Verification items for the finished model (mm, model axes). Face numbers are marked on the shaded views. A direction names the side the tool comes from. Give positions to 0.01 mm unless a question says otherwise; leave off trailing zeros. Order: outer loops, then holes, each group sorted by start corner. A loop starts at its lowest first (then second) coordinate and runs counter-clockwise, first axis right, second up. Notation, with made-up numbers: (-36.5, 56) -> (4.5, 56) arc R22 ccw to (4.5, 83) -> close; hole circle Ø11 at (37, 21.5). An arc over 180 degrees is marked (long way). Write each question's results on one line, items separated by ' | '. Start each with the question number.
1. Cross-section at C-C, the plane y = 0. Enter the section's corners in (x, z) (3 decimals).
2. Mould release check, pull along Y, two halves, no side actions. Record for the marked faces 4, 5 and 6: +Y half, -Y half, draft (parallel to the pull), parting line (faces both ways), or undercut.
3. Material ranges on L1, parallel to Z at x = 6.5, y = 1.75; L2, parallel to X at y = 2.5, z = 3; L3, parallel to X at y = 3, z = 3, recorded low to high. Write a range as from..to.
4. Cross-section at A-A, the plane z = 3. Enter the section's corners in (x, y), then the cut area to 3 significant figures.
5. Set-up check for the marked faces 1, 2 and 3: record each of +Z, -Z, +X, -X, +Y, -Y from which the full face is reachable in a straight line by a thin tool's end or side.
6. Cross-section at B-B, the plane x = 9.5. Enter the section's corners in (y, z).
7. Cross-section at D-D, the plane z = 1. Enter the section's corners in (x, y).
8. Depth check by flat-ended pin: pin 1 Ø1.2 at (y, z) = (0.5, 7) entering from +X (3 decimals); pin 2 Ø3 at (y, z) = (-5.5, 5) entering from +X; pin 3 Ø1.2 at (x, z) = (5.5, 4) entering from -Y; pin 4 Ø1 at (x, z) = (9.5, 3) entering from +Y. Enter the tip coordinate at first touch or a pass-through.
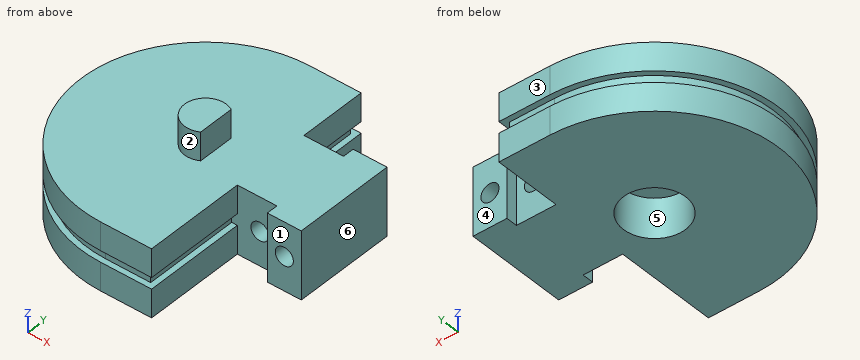
from build123d import *

# Parameters (mm, degrees)
BOSS_EXTRUDE1_DEPTH = 6
CUT_EXTRUDE1_START  = 10
SKETCH2_R           = 0.8
CUT_EXTRUDE1_DEPTH  = 22
CUT_EXTRUDE2_START  = 3
CUT_EXTRUDE2_DEPTH  = 0.5
BOSS_EXTRUDE2_START = 6
BOSS_EXTRUDE2_DEPTH = 2.5
SKETCH5_R           = 2.75
CUT_EXTRUDE3_DEPTH  = 3.5


with BuildPart() as part:
    # Sketch1 → Boss-Extrude1 (new body)
    with BuildSketch(Plane.XY):
        with BuildLine():
            Line((11, 6), (11, -3))
            Line((11, -3), (8, -3))
            Line((8, -3), (8, -2))
            Line((8, -2), (4.5, -2))
            Line((4.5, -2), (4.5, -11))
            Line((4.5, -11), (0, -11))
            ThreePointArc((0, -11), (-11, 0), (0, 11))
            Line((0, 11), (4.5, 11))
            Line((4.5, 11), (4.5, 5))
            Line((4.5, 5), (8, 5))
            Line((8, 5), (8, 6))
            Line((8, 6), (11, 6))
        make_face()
    extrude(amount=BOSS_EXTRUDE1_DEPTH)

    # Sketch2 → Cut-Extrude1 (cut, through all)
    with BuildSketch(Plane(origin=(0, 0, 0), x_dir=(1, 0, 0), z_dir=(0, 1, 0)).offset(CUT_EXTRUDE1_START)):
        with Locations((6.5, -3)):
            Circle(SKETCH2_R)
        with Locations((9.5, -3)):
            Circle(SKETCH2_R)
    extrude(amount=-CUT_EXTRUDE1_DEPTH, mode=Mode.SUBTRACT)

    # Sketch3 → Cut-Extrude2 (cut, symmetric)
    with BuildSketch(Plane.XY.offset(CUT_EXTRUDE2_START)):
        with BuildLine():
            Line((0, 11), (4.5, 11))
            Line((4.5, 11), (4.5, 5))
            Line((4.5, 5), (4, 5))
            Line((4, 5), (4, 10.5))
            Line((4, 10.5), (0, 10.5))
            ThreePointArc((0, 10.5), (-10.5, 0), (0, -10.5))
            Line((0, -10.5), (4, -10.5))
            Line((4, -10.5), (4, -2))
            Line((4, -2), (4.5, -2))
            Line((4.5, -2), (4.5, -11))
            Line((4.5, -11), (0, -11))
            ThreePointArc((0, -11), (-11, 0), (0, 11))
        make_face()
    extrude(amount=CUT_EXTRUDE2_DEPTH, both=True, mode=Mode.SUBTRACT)

    # Sketch4 → Boss-Extrude2 (add)
    with BuildSketch(Plane.XY.offset(BOSS_EXTRUDE2_START)):
        with BuildLine():
            Line((0.925, 1.602146997), (0.925, -1.602146997))
            ThreePointArc((0.925, -1.602146997), (-1.85, 0), (0.925, 1.602146997))
        make_face()
    extrude(amount=BOSS_EXTRUDE2_DEPTH)

    # Sketch5 → Cut-Extrude3 (cut)
    with BuildSketch(Plane.XY):
        Circle(SKETCH5_R)
    extrude(amount=CUT_EXTRUDE3_DEPTH, mode=Mode.SUBTRACT)


solid = part.part
Results below:
1) outline: (-11, 0) -> (-2.75, 0) -> (-2.75, 3.5) -> (2.75, 3.5) -> (2.75, 0) -> (11, 0) -> (11, 6) -> (0.925, 6) -> (0.925, 8.5) -> (-1.85, 8.5) -> (-1.85, 6) -> (-11, 6) -> (-11, 3.5) -> (-10.5, 3.5) -> (-10.5, 2.5) -> (-11, 2.5) -> close; hole circle Ø1.6 at (6.5, 3); hole circle Ø1.6 at (9.5, 3)
2) face 4: +Y half | face 5: undercut | face 6: draft
3) L1: z = 0..2.2, 3.8..6 | L2: x = -10.2..-1.15, 1.15..5.7, 7.3..8.7, 10.3..11 | L3: x = -10.06..5.7, 7.3..8.7, 10.3..11
4) outline: (0, -10.5) -> (4, -10.5) -> (4, -2) -> (5.7, -2) -> (5.7, 5) -> (4, 5) -> (4, 10.5) -> (0, 10.5) arc R10.5 ccw to start; (7.3, -2) -> (8, -2) -> (8, -3) -> (8.7, -3) -> (8.7, 6) -> (8, 6) -> (8, 5) -> (7.3, 5) -> close; (10.3, -3) -> (11, -3) -> (11, 6) -> (10.3, 6) -> close; hole circle Ø5.5 at (0, 0) | area: 263 mm²
5) face 1: +Z, -Z, +X, -Y | face 2: +Z | face 3: +Z, -Z, +X, -X, +Y
6) outline: (-3, 0) -> (6, 0) -> (6, 2.2) -> (-3, 2.2) -> close; (-3, 3.8) -> (6, 3.8) -> (6, 6) -> (-3, 6) -> close
7) outline: (0, -11) -> (4.5, -11) -> (4.5, -2) -> (8, -2) -> (8, -3) -> (11, -3) -> (11, 6) -> (8, 6) -> (8, 5) -> (4.5, 5) -> (4.5, 11) -> (0, 11) arc R11 ccw to start; hole circle Ø5.5 at (0, 0)
8) pin 1: stops at x = 0.925 | pin 2: stops at x = 4.5 | pin 3: stops at y = -2 | pin 4: passes through
